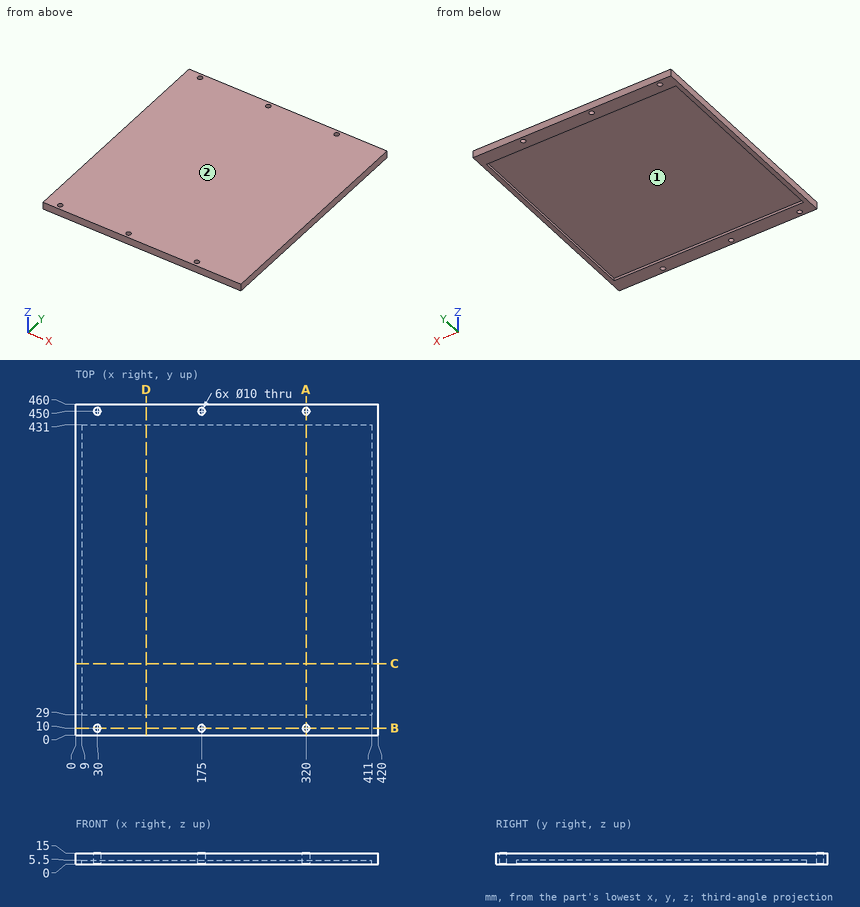
Input: dimensioned drawing with shaded views. Units: mm. Origin: part minimum x, y, z. Coordinates: 2 decimals unless noted, no trailing zeros. Order: outer loops, then holes, each group sorted by start corner. A loop starts at its lowest first (then second) coordinate and runs counter-clockwise, first axis right, second up. Notation, with made-up numbers: (-18.75, 11) - (-6.75, 11) arc R19 cw to (-6.75, 32) - close; hole circle Ø7 at (75.5, 53.25). An arc over 180 degrees is marked (long way). Return JSON: item names as keys, results as strings. Group by question number.
1. Cut plane C-C (y = 99.5). Output: boundary loops of the cut face in (x, z), plus the area to 3 significant figures.
2. Cut plane B-B (y = 10). Output: boundary loops of the cut face in (x, z), plus the area to 3 significant figures.
3. Material intervals for line 1 along X through (y, z) = (450, 10.75); line 2 along Y through (x, z) = (30, 11); line 3 along Y through (x, z) = (320, 5.25), sorted ascending. Write a range as [from, to].
4. Cut plane A-A (x = 320). Output: boundary loops of the cut face in (y, z).
5. Pull-direction query (Y, two-part tool) for the marked faces 1 and 2; classes: pulls with the +Y half, pulls with the -Y half, needs draft (parallel to the pull), parting line crosses it, or undercut.
6. Cut plane D-D (x = 98). Output: boundary loops of the cut face in (y, z).
Resolved:
{
 "1": {"outline": "(0, 0) - (9, 0) - (9, 5.5) - (411, 5.5) - (411, 0) - (420, 0) - (420, 15) - (0, 15) - close", "area": "4,090 mm²"},
 "2": {"outline": "(0, 0) - (25, 0) - (25, 15) - (0, 15) - close; (35, 0) - (170, 0) - (170, 15) - (35, 15) - close; (180, 0) - (315, 0) - (315, 15) - (180, 15) - close; (325, 0) - (420, 0) - (420, 15) - (325, 15) - close", "area": "5,850 mm²"},
 "3": {"line 1": "x = [0, 25], [35, 170], [180, 315], [325, 420]", "line 2": "y = [0, 5], [15, 445], [455, 460]", "line 3": "y = [0, 5], [15, 29], [431, 445], [455, 460]"},
 "4": {"outline": "(0, 0) - (5, 0) - (5, 15) - (0, 15) - close; (15, 0) - (29, 0) - (29, 5.5) - (431, 5.5) - (431, 0) - (445, 0) - (445, 15) - (15, 15) - close; (455, 0) - (460, 0) - (460, 15) - (455, 15) - close"},
 "5": {"face 1": "undercut", "face 2": "needs draft"},
 "6": {"outline": "(0, 0) - (29, 0) - (29, 5.5) - (431, 5.5) - (431, 0) - (460, 0) - (460, 15) - (0, 15) - close"}
}
